```python
from build123d import *

# Parameters (mm, degrees)
BOSS_EXTRUDE1_DEPTH  = 4.7625
M4_CLEARANCE_HOLE1_D = 4.5


with BuildPart() as part:
    # Sketch1 → Boss-Extrude1 (new body)
    with BuildSketch(Plane.XY):
        with BuildLine():
            Line((-94.022602581, 36.539962058), (-94.022602581, 19.178370731))
            ThreePointArc((-94.022602581, 19.178370731), (-93.488675507, 16.852246076), (-91.993785217, 14.99180606))
            Line((-91.993785217, 14.99180606), (-78.162107839, 4.072060761))
            ThreePointArc((-78.162107839, 4.072060761), (-73.397757976, 1.461750489), (-68.040838029, 0.558335853))
            Line((-68.040838029, 0.558335853), (-67.038691488, 0.558335853))
            ThreePointArc((-67.038691488, 0.558335853), (-63.538253204, -0.87137959), (-62.039667189, -4.342891419))
            ThreePointArc((-62.039667189, -4.342891419), (-56.040838029, -10.224364147), (-50.04200887, -4.342891419))
            ThreePointArc((-50.04200887, -4.342891419), (-48.543422854, -0.87137959), (-45.04298457, 0.558335853))
            Line((-45.04298457, 0.558335853), (-7.916602581, 0.558335853))
            Line((-7.916602581, 0.558335853), (4.631523913, -3.09333052))
            ThreePointArc((4.631523913, -3.09333052), (10.550693091, -1.574959819), (12.069063792, 4.344209359))
            Line((12.069063792, 4.344209359), (8.417397419, 16.892335853))
            Line((8.417397419, 16.892335853), (8.417397419, 75.581748009))
            ThreePointArc((8.417397419, 75.581748009), (9.768409389, 79.000064314), (13.091351964, 80.57110612))
            ThreePointArc((13.091351964, 80.57110612), (18.700097419, 86.558335853), (13.091351964, 92.545565587))
            ThreePointArc((13.091351964, 92.545565587), (9.768409389, 94.116607393), (8.417397419, 97.534923698))
            Line((8.417397419, 97.534923698), (8.417397419, 156.224335853))
            Line((8.417397419, 156.224335853), (12.069063792, 168.772462348))
            ThreePointArc((12.069063792, 168.772462348), (10.550693091, 174.691631526), (4.631523913, 176.210002227))
            Line((4.631523913, 176.210002227), (-7.916602581, 172.558335853))
            Line((-7.916602581, 172.558335853), (-45.04298457, 172.558335853))
            ThreePointArc((-45.04298457, 172.558335853), (-48.543422854, 173.988051296), (-50.04200887, 177.459563126))
            ThreePointArc((-50.04200887, 177.459563126), (-56.040838029, 183.341035853), (-62.039667189, 177.459563126))
            ThreePointArc((-62.039667189, 177.459563126), (-63.538253204, 173.988051296), (-67.038691488, 172.558335853))
            Line((-67.038691488, 172.558335853), (-68.040838029, 172.558335853))
            ThreePointArc((-68.040838029, 172.558335853), (-73.397757976, 171.654921218), (-78.162107839, 169.044610946))
            Line((-78.162107839, 169.044610946), (-91.993785217, 158.124865647))
            ThreePointArc((-91.993785217, 158.124865647), (-93.488675507, 156.264425631), (-94.022602581, 153.938300976))
            Line((-94.022602581, 153.938300976), (-94.022602581, 136.576709649))
            ThreePointArc((-94.022602581, 136.576709649), (-95.487068676, 133.041175743), (-99.022602581, 131.576709649))
            Line((-99.022602581, 131.576709649), (-99.522602581, 131.576709649))
            ThreePointArc((-99.522602581, 131.576709649), (-105.522602581, 125.576709649), (-99.522602581, 119.576709649))
            Line((-99.522602581, 119.576709649), (-99.022602581, 119.576709649))
            ThreePointArc((-99.022602581, 119.576709649), (-95.487068676, 118.112243554), (-94.022602581, 114.576709649))
            Line((-94.022602581, 114.576709649), (-94.022602581, 58.539962058))
            ThreePointArc((-94.022602581, 58.539962058), (-95.487068676, 55.004428152), (-99.022602581, 53.539962058))
            Line((-99.022602581, 53.539962058), (-99.522602581, 53.539962058))
            ThreePointArc((-99.522602581, 53.539962058), (-105.522602581, 47.539962058), (-99.522602581, 41.539962058))
            Line((-99.522602581, 41.539962058), (-99.022602581, 41.539962058))
            ThreePointArc((-99.022602581, 41.539962058), (-95.487068676, 40.075495964), (-94.022602581, 36.539962058))
        make_face()
    extrude(amount=-BOSS_EXTRUDE1_DEPTH)

    # M4 Clearance Hole1 (through all)
    with Locations(Plane(origin=(0, 0, -4.7625), x_dir=(-1, 0, 0), z_dir=(0, 0, -1))):
        with Locations((-12.700097419, 86.558335853), (-6.308052404, 2.667680868), (-6.308052404, 170.448990839), (99.522602581, 47.539962058), (99.522602581, 125.576709649), (56.040838029, 177.341035853), (56.040838029, -4.224364147)):
            Hole(M4_CLEARANCE_HOLE1_D / 2)


solid = part.part
```
Design review of the part built by this model. Coordinates are the model's own, in mm. A direction names the side the tool comes from. Give positions to 0.01 mm unless a question says otherwise; leave off trailing zeros. Loops run counter-clockwise (first coordinate to the right, second up) from the corner with the lowest first, then second, coordinate; pieces in that order, holes last. Notation, with made-up numbers: (40.5, 40.25) -> (60.5, 40.25) arc R19 ccw to (60.5, 53.25) -> close; hole circle Ø4 at (4, -27.75). An arc over 180 degrees is marked (long way). One line per item, written item: value.
Q1. We need section B-B on z = -2.6. Give the number of separate pieces and of enclosed holes in the cut face, and give its area (3 significant figures).
Numbers:
separate pieces: 1
enclosed holes: 7
area: 18,000 mm^2
Q2. Draft analysis for pull direction X (two halves, no side actions). For faces 1 (the flat face through (-44, 88, -4.762)), 2 (the cylindrical face through (14.78, 85.7, -2.35)), 3 (the cylindrical face through (9.73, 78.96, -2.35)), state which applies: pulls with the +X half, pulls with the -X half, needs draft (parallel to the pull), parting line crosses it, or undercut.
Numbers:
face 1: needs draft
face 2: undercut
face 3: pulls with the +X half
Q3. Machinability: for faces 4 (the flat face through (-94.023, 87, -2)), 5 (the flat face through (-1.55, 174.41, -2.35)), 6 (the cylindrical face through (6.02, 4.9, -2.35)), 7 (the flat face through (8.417, 46, -2)), which of the approach directions +Z, -Z, +X, -X, +Y, -Y give a long, thin tool a straight path to every point of the face, cutting with its end or side? Answer none if there is none.
Numbers:
face 4: +Z, -Z, -X
face 5: +Z, -Z, +Y
face 6: +Z, -Z
face 7: +Z, -Z, +X
Q4. We need section A-A on x = -32.5. Give the boundary of the cut face in (y, z).
Numbers:
outline: (0.56, -4.76) -> (172.56, -4.76) -> (172.56, 0) -> (0.56, 0) -> close
Q5. We need section C-C on y = 25.5. Give the boundary of the cut face in (x, z), and give its area (3 significant figures).
Numbers:
outline: (-94.02, -4.76) -> (8.42, -4.76) -> (8.42, 0) -> (-94.02, 0) -> close
area: 488 mm^2
Q6. For L1, parallel to Y at x = -54, z = -0.9; L2, parallel to X at y = 72.5, z = -0.3; L3, parallel to Y at x = 7.5, z = -1.95, list the stretches that pass through material, from the lowest coordinate up.
Numbers:
L1: y = -9.87 to -5.17, -3.28 to 176.39, 178.29 to 182.98
L2: x = -94.02 to 8.42
L3: y = -3.21 to 0.76, 4.58 to 168.54, 172.36 to 176.33
Q7. For pin 1 Ø2.5 at (x, z) = (-32.5, -2) entering from -Y; pin 2 Ø2 at (y, z) = (116, -4) entering from -X; pin 3 Ø2 at (y, z) = (144, -2.5) entering from +X; pin 4 Ø4 at (x, y) = (6.31, 2.67) entering from -Z, all flat-tipped, find the tip position at first contact; note any pin that passes through.
Numbers:
pin 1: stops at y = 0.56
pin 2: stops at x = -94.65
pin 3: stops at x = 8.42
pin 4: passes through
